from build123d import *

# Parameters (mm, degrees)
CROQUIS1_R              = 13
CROQUIS1_R_2            = 5
SALIENTE_EXTRUIR1_DEPTH = 8
CROQUIS2_R              = 11
CROQUIS2_R_2            = 6.25
CORTAR_EXTRUIR1_DEPTH   = 0.1
CORTAR_EXTRUIR2_START   = -0.1
CROQUIS3_R              = 11
CROQUIS3_R_2            = 6.25
CORTAR_EXTRUIR2_DEPTH   = 0.1


with BuildPart() as part:
    # Croquis1 → Saliente-Extruir1 (new body)
    with BuildSketch(Plane.XY):
        Circle(CROQUIS1_R)
        Circle(CROQUIS1_R_2, mode=Mode.SUBTRACT)
    extrude(amount=SALIENTE_EXTRUIR1_DEPTH)

    # Croquis2 → Cortar-Extruir1 (cut)
    with BuildSketch(Plane.XY.offset(8)):
        Circle(CROQUIS2_R)
        Circle(CROQUIS2_R_2, mode=Mode.SUBTRACT)
    extrude(amount=-CORTAR_EXTRUIR1_DEPTH, mode=Mode.SUBTRACT)

    # Croquis3 → Cortar-Extruir2 (cut)
    with BuildSketch(Plane(origin=(0, 0, 0), x_dir=(-1, 0, 0), z_dir=(0, 0, -1)).offset(CORTAR_EXTRUIR2_START)):
        with Locations(Location((0, 0, 0), (0, 0, 180))):
            Circle(CROQUIS3_R)
        with Locations(Location((0, 0, 0), (0, 0, 180))):
            Circle(CROQUIS3_R_2, mode=Mode.SUBTRACT)
    extrude(amount=CORTAR_EXTRUIR2_DEPTH, mode=Mode.SUBTRACT)


solid = part.part
For this review, take the finished solid that the model builds, in its own axes (mm). A direction names the side the tool comes from. Give positions to 0.01 mm unless a question says otherwise; leave off trailing zeros. Loops run counter-clockwise (first coordinate to the right, second up) from the corner with the lowest first, then second, coordinate; pieces in that order, holes last. Notation, with made-up numbers: M 44.25,-26 L 53.25,-26 A27 cw 53.25,4 Z; hole C 27,50.5 d6. An arc over 180 degrees is marked long. Put each result on its own line as item: value. Start each with the question number.
(1) Machinability: for faces 1 (the flat face through (5, -5, 7.9)), 2 (the flat face through (2, 5, 8)), which of the approach directions +Z, -Z, +X, -X, +Y, -Y give a long, thin tool a straight path to every point of the face, cutting with its end or side? Answer none if there is none.
(2) Add section A-A, the plane x = 0. Write out the cut boundary in (y, z), then the cut area to 3 significant figures.
(3) Add section D-D, the plane z = 6. Write out the cut boundary in (x, y), then the cut area to 3 significant figures.
(4) Wall thickness on L1, parallel to Y at x = 0, z = 0.05; L2, parallel to Y at x = 0, z = 2; L3, parallel to Z at x = -6.75, y = -8: over which ranges is each line inside the solid? List them lowest first.
(5) The part is to be moulded in two halves that separate along Y. For faces 3 (the flat face through (-11, 3, 8)), 4 (the flat face through (5, 5, 0.1)), 5 (the cylindrical face through (-10.316, -7.91, 3.944)), say which applies: +Y half, -Y half, draft (parallel to the pull), parting line (faces both ways), or undercut.
(6) Add section C-C, the plane y = -8.5. Write out the cut boundary in (x, z), then the cut area to 3 significant figures.
(7) For pin 1 (3 mm diameter, centred on x = -9.5, z = 2, fed in from +Y); pin 2 (1 mm diameter, centred on x = 1, z = 4.5, fed in from +Y); pin 3 (3 mm diameter, centred on x = -8, z = 6, fed in from -Y), all flat-tipped, find the tip position at first contact; note any pin that passes through.
Result:
1. face 1: +Z
1. face 2: +Z, +X, -X, +Y, -Y
2. outline: M -13,0 L -11,0 L -11,0.1 L -6.25,0.1 L -6.25,0 L -5,0 L -5,8 L -6.25,8 L -6.25,7.9 L -11,7.9 L -11,8 L -13,8 Z; M 5,0 L 6.25,0 L 6.25,0.1 L 11,0.1 L 11,0 L 13,0 L 13,8 L 11,8 L 11,7.9 L 6.25,7.9 L 6.25,8 L 5,8 Z
2. area: 126 mm^2
3. outline: C 0,0 d26; hole C 0,0 d10
3. area: 452 mm^2
4. L1: y = -13 to -11, -6.25 to -5, 5 to 6.25, 11 to 13
4. L2: y = -13 to -5, 5 to 13
4. L3: z = 0.1 to 7.9
5. face 3: draft
5. face 4: undercut
5. face 5: parting line
6. outline: M -9.84,0 L -6.98,0 L -6.98,0.1 L 6.98,0.1 L 6.98,0 L 9.84,0 L 9.84,8 L 6.98,8 L 6.98,7.9 L -6.98,7.9 L -6.98,8 L -9.84,8 Z
6. area: 155 mm^2
7. pin 1: stops at y = 10.25
7. pin 2: stops at y = 12.99
7. pin 3: stops at y = -11.26
